For this review, take the finished solid that the model builds, in its own axes (mm). Face numbers are marked on the shaded views. A direction names the side the tool comes from. Give positions to 0.01 mm unless a question says otherwise; leave off trailing zeros. Loops run counter-clockwise (first coordinate to the right, second up) from the corner with the lowest first, then second, coordinate; pieces in that order, holes last. Notation, with made-up numbers: (62.25, -21) -> (85.25, -21) arc R29 cw to (85.25, 18) -> close; hole circle Ø5 at (74.5, 31). An arc over 180 degrees is marked (long way). One line per question, with ' | ' between items. Start each with the question number.
(1) Draft analysis for pull direction Y (two halves, no side actions). For the marked faces 3, 4 and 5, state which applies: +Y half, -Y half, draft (parallel to the pull), parting line (faces both ways), or undercut.
(2) Wall thickness on probe 1 along Y at (x, z) = (0, -1.2); probe 2 along Y at (x, z) = (0, 8.25); probe 3 along Z at (x, y) = (-1.5, -2.25): over which ranges is each line inside the solid? List them lowest first.
(3) Consider section A-A (x = 0). Write out the cut boundary in (y, z).
(4) Consider section C-C (z = 13). Write out the cut boundary in (x, y).
(5) Insertion check: P1, Ø6.5, axis at x = -1, y = 0.5, coming from the -Z side; P2, Ø6, axis at x = -5.5, z = 0.5, coming from the -Y side; P3, Ø10, axis at y = 5.5, z = 2, coming from the -X side. Each pin has a flat end and moves straight along its axis. Give the tip position at first contact, or say it passes through.
(6) Consider section B-B (z = 3). Write out the cut boundary in (x, y), and give its area (3 significant figures).
(7) Tool access review of the marked faces 1 and 2: name each direction out of +Z, -Z, +X, -X, +Y, -Y from which nothing blocks a thin tool from reaching the whole face with its end or side.
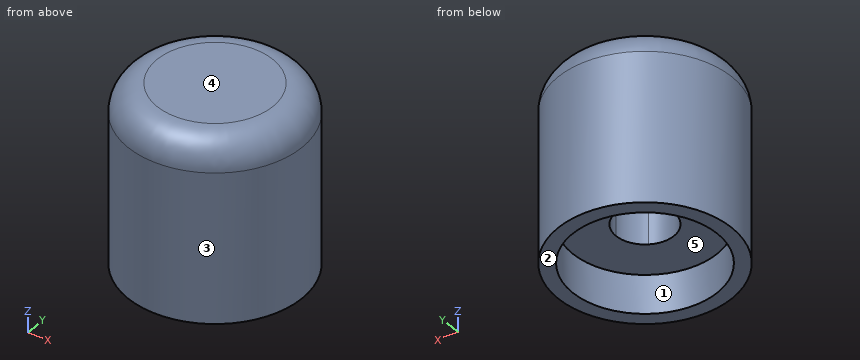
from build123d import *

# Parameters (mm, degrees)
F0_R     = 9
F0_R_2   = 7.5
F1_DEPTH = 14.5
F2_DEPTH = 12
F3_DEPTH = 4
F4_R     = 3


with BuildPart() as f1:
    # F0 (on Top) → F1 (new body)
    with BuildSketch(Plane.XY):
        Circle(F0_R)
        Circle(F0_R_2, mode=Mode.SUBTRACT)
        Circle(F0_R_2)
        with BuildLine():
            ThreePointArc((1.5, 2.5980762114), (2.5980762114, 1.5), (3, 0))
            ThreePointArc((3, 0), (2.5980762114, -1.5), (1.5, -2.5980762114))
            ThreePointArc((1.5, -2.5980762114), (-3, 0), (1.5, 2.5980762114))
        make_face(mode=Mode.SUBTRACT)
        with BuildLine():
            Line((1.5, -2.5980762114), (1.5, 2.5980762114))
            ThreePointArc((1.5, 2.5980762114), (-3, 0), (1.5, -2.5980762114))
        make_face()
        with BuildLine():
            ThreePointArc((1.5, -2.5980762114), (2.5980762114, -1.5), (3, 0))
            ThreePointArc((3, 0), (2.5980762114, 1.5), (1.5, 2.5980762114))
            Line((1.5, 2.5980762114), (1.5, -2.5980762114))
        make_face()
    extrude(amount=F1_DEPTH)

    # F0 (on Top) → F2 (cut)
    with BuildSketch(Plane.XY):
        with BuildLine():
            Line((1.5, -2.5980762114), (1.5, 2.5980762114))
            ThreePointArc((1.5, 2.5980762114), (-3, 0), (1.5, -2.5980762114))
        make_face()
        with BuildLine():
            ThreePointArc((1.5, -2.5980762114), (2.5980762114, -1.5), (3, 0))
            ThreePointArc((3, 0), (2.5980762114, 1.5), (1.5, 2.5980762114))
            Line((1.5, 2.5980762114), (1.5, -2.5980762114))
        make_face()
    extrude(amount=F2_DEPTH, mode=Mode.SUBTRACT)

    # F0 (on Top) → F3 (join)
    with BuildSketch(Plane.XY):
        Circle(F0_R)
        Circle(F0_R_2, mode=Mode.SUBTRACT)
    extrude(amount=-F3_DEPTH)

    # F4
    f4_edges = [f1.edges().sort_by_distance(p)[0] for p in [
        (-9, 0, 14.5),
    ]]
    fillet(f4_edges, radius=F4_R)


solid = f1.part
A:
1) face 3: parting line | face 4: draft | face 5: undercut
2) probe 1: y = -9 to -7.5, 7.5 to 9 | probe 2: y = -9 to -3, 3 to 9 | probe 3: z = 12 to 14.5
3) outline: (-9, -4) -> (-7.5, -4) -> (-7.5, 0) -> (-3, 0) -> (-3, 12) -> (3, 12) -> (3, 0) -> (7.5, 0) -> (7.5, -4) -> (9, -4) -> (9, 11.5) arc R3 ccw to (6, 14.5) -> (-6, 14.5) arc R3 ccw to (-9, 11.5) -> close
4) outline: circle Ø17.2 at (0, 0)
5) P1: stops at z = 0 | P2: stops at y = -8.65 | P3: stops at x = -8.99
6) outline: circle Ø18 at (0, 0); hole circle Ø6 at (0, 0) | area: 226 mm^2
7) face 1: -Z | face 2: -Z, +X, -X, +Y, -Y
